Geometry check sheet. Reference: the model listing, model coordinates, mm. Face numbers are marked on the shaded views. A direction names the side the tool comes from. Give positions to 0.01 mm unless a question says otherwise; leave off trailing zeros. Loops run counter-clockwise (first coordinate to the right, second up) from the corner with the lowest first, then second, coordinate; pieces in that order, holes last. Notation, with made-up numbers: (6, 23.25) -> (62, 23.25) arc R19 ccw to (62, 53.25) -> close; hole circle Ø4 at (-17.75, 29). An arc over 180 degrees is marked (long way). One line per item, written item: value. Start each with the question number.
(1) Sectioned sample at C-C, the plane z = -33. Record the cut outline in (x, y).
(2) Sectioned sample at D-D, the plane y = 29. Record the cut outline in (x, z), then the cut area to 3 significant figures.
(3) Sectioned sample at B-B, the plane x = 41. Record the cut outline in (y, z), then the cut area to 3 significant figures.
(4) Draft check along Y on the marked faces 1, 2 and 3. Enter one of: pulls with the +Y half, pulls with the -Y half, needs draft (parallel to the pull), parting line crosses it, or undercut.
(5) Gauge pin test, flat ends, axial feed: pin 1 Ø4 at (y, z) = (5, -4.5) entering from +X; pin 2 Ø8 at (y, z) = (8, -24) entering from -X; pin 3 Ø10 at (y, z) = (24.5, -20.5) entering from +X; pin 4 Ø9 at (x, y) = (10, 31) entering from +Z. Record the tip position at first contact, or that the pin passes through.
(6) Tool access check on the marked faces 4, 5, 6 and 7. Record the directions out of +Z, -Z, +X, -X, +Y, -Y that give a thin tool (end or side, any length) a straight path to the whole face; none if there is none.
(7) Scan lines: line 1 along Y through (x, z) = (10, -2); line 2 along Y through (x, z) = (85, -11); line 3 along X through (y, z) = (4, -23.5). Record each from-to range of solid material in increasing order. Write a range as from..to.
(8) Sectioned sample at A-A, the plane x = 10. Record the cut outline in (y, z).
from build123d import *

# Parameters (mm, degrees)
BOSS_EXTRUDE1_DEPTH = 16
FILLET1_R           = 2
SKETCH3_R           = 5
BOSS_EXTRUDE2_DEPTH = 10
LPATTERN1_COUNT     = 2
LPATTERN1_PITCH     = 30
SKETCH4_R           = 5
BOSS_EXTRUDE3_DEPTH = 45


with BuildPart() as part:
    # Sketch2 → Boss-Extrude1 (new body)
    with BuildSketch(Plane(origin=(0, 0, 0), x_dir=(1, 0, 0), z_dir=(0, 1, 0))):
        Polygon((0, 30), (0, 40), (90, 40), (90, 28), (120, 28), (120, 12), (90, 12), (90, 0), (0, 0), (0, 10), (70, 10), (70, 30), align=None)
    extrude(amount=BOSS_EXTRUDE1_DEPTH)

    # Fillet1
    fillet1_edges = [part.edges().sort_by_distance(p)[0] for p in [
        (105, 16, -12),
        (105, 0, -28),
        (105, 0, -12),
        (105, 16, -28),
    ]]
    fillet(fillet1_edges, radius=FILLET1_R)

    # Sketch3 → Boss-Extrude2 (add)
    with BuildSketch(Plane.XY):
        with BuildLine():
            Line((0, 16), (20, 16))
            Line((20, 16), (20, 31))
            ThreePointArc((20, 31), (10, 41), (0, 31))
            Line((0, 31), (0, 16))
        make_face()
        with Locations((10, 31)):
            Circle(SKETCH3_R, mode=Mode.SUBTRACT)
    boss_extrude2 = extrude(amount=-BOSS_EXTRUDE2_DEPTH)

    # LPattern1: Boss-Extrude2 ×2
    with Locations(*[(0, 0, -i * LPATTERN1_PITCH) for i in range(1, LPATTERN1_COUNT)]):
        add(boss_extrude2)

    # Sketch4 → Boss-Extrude3 (add)
    with BuildSketch(Plane(origin=(0, 16, 0), x_dir=(1, 0, 0), z_dir=(0, 1, 0))):
        with Locations((80, 20)):
            Circle(SKETCH4_R)
    extrude(amount=BOSS_EXTRUDE3_DEPTH)


solid = part.part
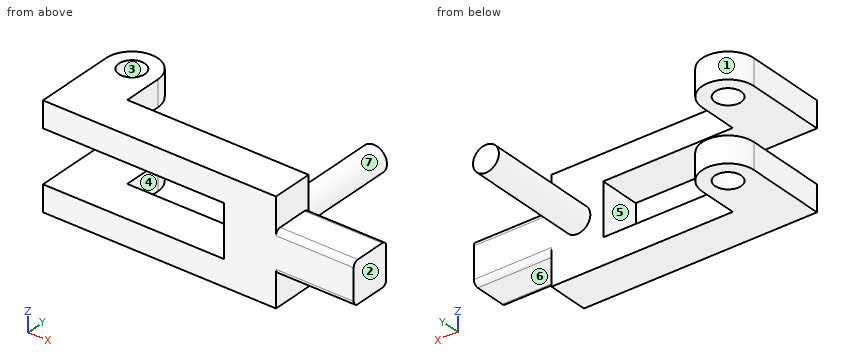
Calculated:
1. outline: (0, 0) -> (90, 0) -> (90, 16) -> (20, 16) -> (20, 31) arc R10 ccw to (0, 31) -> close; hole circle Ø10 at (10, 31)
2. outline: (0, -40) -> (5.42, -40) -> (5.42, -30) -> (0, -30) -> close; (0, -10) -> (5.42, -10) -> (5.42, 0) -> (0, 0) -> close; (14.58, -40) -> (20, -40) -> (20, -30) -> (14.58, -30) -> close; (14.58, -10) -> (20, -10) -> (20, 0) -> (14.58, 0) -> close; circle Ø10 at (80, -20)
2. area: 295 mm2
3. outline: (0, -40) -> (16, -40) -> (16, -30) -> (0, -30) -> close; (0, -10) -> (16, -10) -> (16, 0) -> (0, 0) -> close
3. area: 320 mm2
4. face 1: pulls with the +Y half
4. face 2: needs draft
4. face 3: undercut
5. pin 1: stops at x = 90
5. pin 2: stops at x = 70
5. pin 3: stops at x = 85
5. pin 4: passes through
6. face 4: +Z, -Z, +X, +Y
6. face 5: -X, +Y, -Y
6. face 6: -Z, +X, +Y, -Y
6. face 7: +Y
7. line 1: y = 0..26, 36..41
7. line 2: y = 0..16
7. line 3: x = 70..120
8. outline: (0, -40) -> (26, -40) -> (26, -30) -> (0, -30) -> close; (0, -10) -> (26, -10) -> (26, 0) -> (0, 0) -> close; (36, -40) -> (41, -40) -> (41, -30) -> (36, -30) -> close; (36, -10) -> (41, -10) -> (41, 0) -> (36, 0) -> close
